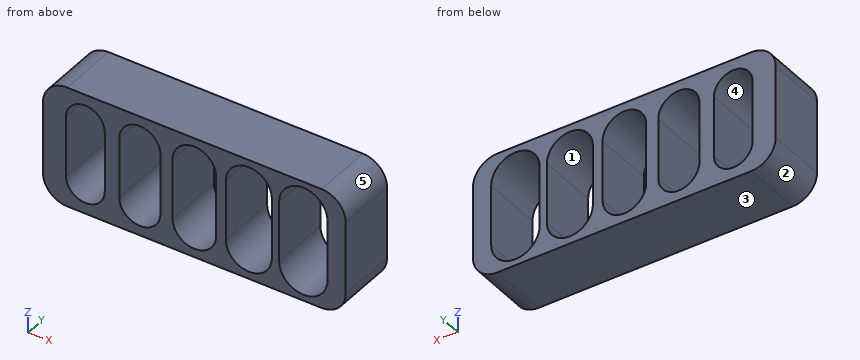
from build123d import *

# Parameters (mm, degrees)
SKETCH1_W           = 25
SKETCH1_H           = 10
BOSS_EXTRUDE1_DEPTH = 5
FILLET1_R           = 2


with BuildPart() as part:
    # Sketch1 → Boss-Extrude1 (new body)
    with BuildSketch(Plane(origin=(0, 0, 0), x_dir=(1, 0, 0), z_dir=(0, 1, 0))):
        Rectangle(SKETCH1_W, SKETCH1_H)
        with BuildLine():
            Line((-1.8, -2.5), (-1.8, 2.5))
            ThreePointArc((-1.8, 2.5), (0, 4.3), (1.8, 2.5))
            Line((1.8, 2.5), (1.8, -2.5))
            ThreePointArc((1.8, -2.5), (0, -4.3), (-1.8, -2.5))
        make_face(mode=Mode.SUBTRACT)
        with BuildLine():
            Line((-6.2, -2.5), (-6.2, 2.5))
            ThreePointArc((-6.2, 2.5), (-4.5, 4.2), (-2.8, 2.5))
            Line((-2.8, 2.5), (-2.8, -2.5))
            ThreePointArc((-2.8, -2.5), (-4.5, -4.2), (-6.2, -2.5))
        make_face(mode=Mode.SUBTRACT)
        with BuildLine():
            Line((-10.6, -2.5), (-10.6, 2.5))
            ThreePointArc((-10.6, 2.5), (-9, 4.1), (-7.4, 2.5))
            Line((-7.4, 2.5), (-7.4, -2.5))
            ThreePointArc((-7.4, -2.5), (-9, -4.1), (-10.6, -2.5))
        make_face(mode=Mode.SUBTRACT)
        with BuildLine():
            Line((2.6, -2.5), (2.6, 2.5))
            ThreePointArc((2.6, 2.5), (4.5, 4.4), (6.4, 2.5))
            Line((6.4, 2.5), (6.4, -2.5))
            ThreePointArc((6.4, -2.5), (4.5, -4.4), (2.6, -2.5))
        make_face(mode=Mode.SUBTRACT)
        with BuildLine():
            Line((7, -2.5), (7, 2.5))
            ThreePointArc((7, 2.5), (9, 4.5), (11, 2.5))
            Line((11, 2.5), (11, -2.5))
            ThreePointArc((11, -2.5), (9, -4.5), (7, -2.5))
        make_face(mode=Mode.SUBTRACT)
    extrude(amount=BOSS_EXTRUDE1_DEPTH)

    # Fillet1
    fillet1_edges = [part.edges().sort_by_distance(p)[0] for p in [
        (-12.5, 2.5, -5),
        (12.5, 2.5, -5),
        (12.5, 2.5, 5),
        (-12.5, 2.5, 5),
    ]]
    fillet(fillet1_edges, radius=FILLET1_R)


solid = part.part
Part model, mm, in its own coordinate system. Face numbers are marked on the shaded views. A direction names the side the tool comes from. Give positions to 0.01 mm unless a question says otherwise; leave off trailing zeros. Order: outer loops, then holes, each group sorted by start corner. A loop starts at its lowest first (then second) coordinate and runs counter-clockwise, first axis right, second up. Notation, with made-up numbers: (37.5, 42) -> (55.5, 42) arc R22 ccw to (55.5, 75) -> close; hole circle Ø7 at (-28.5, 10). An arc over 180 degrees is marked (long way). Use one line per item in the form item = value.
(1) Pull direction Z, two halves, no side cores. Call the marked faces 3, 4 and 5: +Z half, -Z half, draft (parallel to the pull), parting line (faces both ways), or undercut.
Solution:
face_3 = -Z half
face_4 = undercut
face_5 = +Z half
(2) Saw through at B-B (y = 4.5). Write the cut outline in (x, z), then the cut area to 3 significant figures.
Solution:
outline = (-12.5, -3) arc R2 ccw to (-10.5, -5) -> (10.5, -5) arc R2 ccw to (12.5, -3) -> (12.5, 3) arc R2 ccw to (10.5, 5) -> (-10.5, 5) arc R2 ccw to (-12.5, 3) -> close; hole (-10.6, -2.5) arc R1.6 ccw to (-7.4, -2.5) -> (-7.4, 2.5) arc R1.6 ccw to (-10.6, 2.5) -> close; hole (-6.2, -2.5) arc R1.7 ccw to (-2.8, -2.5) -> (-2.8, 2.5) arc R1.7 ccw to (-6.2, 2.5) -> close; hole (-1.8, -2.5) arc R1.8 ccw to (1.8, -2.5) -> (1.8, 2.5) arc R1.8 ccw to (-1.8, 2.5) -> close; hole (2.6, -2.5) arc R1.9 ccw to (6.4, -2.5) -> (6.4, 2.5) arc R1.9 ccw to (2.6, 2.5) -> close; hole (7, -2.5) arc R2 ccw to (11, -2.5) -> (11, 2.5) arc R2 ccw to (7, 2.5) -> close
area = 105 mm²
(3) Saw through at D-D (x = -4.5). Write the cut outline in (y, z).
Solution:
outline = (0, -5) -> (5, -5) -> (5, -4.2) -> (0, -4.2) -> close; (0, 4.2) -> (5, 4.2) -> (5, 5) -> (0, 5) -> close
(4) Tool access for the marked faces 1 and 2: list every direction of +Z, -Z, +X, -X, +Y, -Y with a clear straight run to the whole face (end or side of a thin tool).
Solution:
face_1 = +Y, -Y
face_2 = -Z, -X, +Y, -Y
(5) Saw through at A-A (x = 9). Write the cut outline in (y, z), then the cut area to 3 significant figures.
Solution:
outline = (0, -5) -> (5, -5) -> (5, -4.5) -> (0, -4.5) -> close; (0, 4.5) -> (5, 4.5) -> (5, 5) -> (0, 5) -> close
area = 5.00 mm²
(6) Drill centre lines: line 1 (X direction, y = 4.2, z = -0.75); line 2 (X direction, y = 1.65, z = -3.5); line 3 (Z direction, x = 9.5, y = 4). Where is each one in solid material? Low to high. Write a range as from..to.
Solution:
line_1 = -12.5..-10.6, -7.4..-6.2, -2.8..-1.8, 1.8..2.6, 6.4..7, 11..12.5
line_2 = -12.44..-10.25, -7.75..-5.87, -3.13..-1.5, 1.5..2.88, 6.12..7.27, 10.73..12.44
line_3 = -5..-4.44, 4.44..5
(7) Saw through at C-C (z = 2.25). Write the cut outline in (x, y), then the cut area to 3 significant figures.
Solution:
outline = (-12.5, 0) -> (-10.6, 0) -> (-10.6, 5) -> (-12.5, 5) -> close; (-7.4, 0) -> (-6.2, 0) -> (-6.2, 5) -> (-7.4, 5) -> close; (-2.8, 0) -> (-1.8, 0) -> (-1.8, 5) -> (-2.8, 5) -> close; (1.8, 0) -> (2.6, 0) -> (2.6, 5) -> (1.8, 5) -> close; (6.4, 0) -> (7, 0) -> (7, 5) -> (6.4, 5) -> close; (11, 0) -> (12.5, 0) -> (12.5, 5) -> (11, 5) -> close
area = 35.0 mm²
